Geometry: final body of the model. Coordinates: model frame, mm. A direction names the side the tool comes from. Coordinates: 2 decimals unless noted, no trailing zeros. Order: outer loops, then holes, each group sorted by start corner. A loop starts at its lowest first (then second) coordinate and runs counter-clockwise, first axis right, second up. Notation, with made-up numbers: M 62,0.25 L 72,0.25 A19 ccw 72,14.25 Z; hole C 31,40 d6. An arc over 180 degrees is marked long. One line per question, with ' | ' between items.
from build123d import *

# Parameters (mm, degrees)
SKETCH2_R                 = 23.5
SKETCH2_R_2               = 97
BOSS_EXTRUDE5_DEPTH       = 32
SKETCH3_R                 = 140
SKETCH3_R_2               = 97
BOSS_EXTRUDE8_DEPTH       = 112.5
BOSS_EXTRUDE10_REACH      = 527.627
BOSS_EXTRUDE10_END_RADIUS = 140
SKETCH4_R                 = 100
SKETCH5_R                 = 50
CUT_EXTRUDE1_DEPTH        = 25.5
SKETCH7_R                 = 28.1
CUT_EXTRUDE2_DEPTH        = 328.5
SKETCH9_R                 = 9.714368659
CUT_EXTRUDE3_DEPTH        = 10.5


with BuildPart() as part:
    # Sketch2 → Boss-Extrude5 (new body)
    with BuildSketch(Plane(origin=(0, 0, 0), x_dir=(1, 0, 0), z_dir=(0, 1, 0))):
        with BuildLine():
            ThreePointArc((49.230976904, 178.339293487), (-0.769023096, 228.339293487), (-50.769023096, 178.339293487))
            Line((-50.769023096, 178.339293487), (-50.769023096, 130.470327254))
            ThreePointArc((-50.769023096, 130.470327254), (-121.653121624, 69.285770538), (-138.115414376, -22.893936133))
            Line((-138.115414376, -22.893936133), (-179.061847104, -46.534370091))
            ThreePointArc((-179.061847104, -46.534370091), (-197.363117294, -114.835640281), (-129.061847104, -133.13691047))
            Line((-129.061847104, -133.13691047), (-87.606106294, -109.202427354))
            ThreePointArc((-87.606106294, -109.202427354), (0.823323405, -139.997579045), (88.884437472, -108.164489437))
            Line((88.884437472, -108.164489437), (129.8308702, -131.804923395))
            ThreePointArc((129.8308702, -131.804923395), (198.13214039, -113.503653206), (179.8308702, -45.202383017))
            Line((179.8308702, -45.202383017), (138.37512939, -21.267899901))
            ThreePointArc((138.37512939, -21.267899901), (120.829798219, 70.711808507), (49.230976904, 131.058425571))
            Line((49.230976904, 131.058425571), (49.230976904, 178.339293487))
        make_face()
        with Locations(Location((-0.769023096, 178.339293487, 0), (0, 0, 270))):
            Circle(SKETCH2_R, mode=Mode.SUBTRACT)
        with Locations(Location((0, 0, 0), (0, 0, 270))):
            Circle(SKETCH2_R_2, mode=Mode.SUBTRACT)
        with Locations(Location((-154.061847104, -89.835640281, 0), (0, 0, 270))):
            Circle(SKETCH2_R, mode=Mode.SUBTRACT)
        with Locations(Location((154.8308702, -88.503653206, 0), (0, 0, 270))):
            Circle(SKETCH2_R, mode=Mode.SUBTRACT)
    extrude(amount=BOSS_EXTRUDE5_DEPTH)

    # Sketch3 → Boss-Extrude8 (add)
    with BuildSketch(Plane(origin=(0, 32, 0), x_dir=(1, 0, 0), z_dir=(0, 1, 0))):
        with Locations(Location((0, 0, 0), (0, 0, 69.411740358))):
            Circle(SKETCH3_R)
        with Locations(Location((0, 0, 0), (0, 0, 270))):
            Circle(SKETCH3_R_2, mode=Mode.SUBTRACT)
    extrude(amount=BOSS_EXTRUDE8_DEPTH)

    # Mirror1: part across plane


with BuildPart() as part_1:
    add(part.part)
    add(part.part.mirror(Plane.ZX.offset(144.5)))

    # Boss-Extrude10: up to this cylinder (the profile starts outside it)
    boss_extrude10_end = Plane(origin=(0, 150.900402, 0), z_dir=(0, -1, 0)) * Cylinder(BOSS_EXTRUDE10_END_RADIUS, 1336.254, mode=Mode.PRIVATE)
    # Sketch4 → Boss-Extrude10 (add, up to the surface)
    with BuildSketch(Plane.XY.offset(160), mode=Mode.PRIVATE) as boss_extrude10_sk1:
        with Locations((0, 150.900402454)):
            Circle(SKETCH4_R)
    boss_extrude10_tool1 = extrude(boss_extrude10_sk1.sketch, amount=-BOSS_EXTRUDE10_REACH, mode=Mode.PRIVATE) - boss_extrude10_end
    add(boss_extrude10_tool1.solids().sort_by_distance((0, 150.900402, 160))[0])

    # Sketch5 → Cut-Extrude1 (cut)
    with BuildSketch(Plane.XY.offset(160)):
        with Locations((0, 150.900402454)):
            Circle(SKETCH5_R)
    extrude(amount=-CUT_EXTRUDE1_DEPTH, mode=Mode.SUBTRACT)

    # Sketch7 → Cut-Extrude2 (cut)
    with BuildSketch(Plane.XY.offset(134.5)):
        with Locations(Location((0, 150.900402454, 0), (0, 0, 90))):
            Circle(SKETCH7_R)
    extrude(amount=-CUT_EXTRUDE2_DEPTH, mode=Mode.SUBTRACT)

    # Sketch9 → Cut-Extrude3 (cut)
    with BuildSketch(Plane.XY.offset(160)):
        with Locations((0, 226.895659714)):
            Circle(SKETCH9_R)
        with Locations((65.813823354, 112.902773824)):
            Circle(SKETCH9_R)
        with Locations((-65.813823354, 112.902773824)):
            Circle(SKETCH9_R)
    extrude(amount=-CUT_EXTRUDE3_DEPTH, mode=Mode.SUBTRACT)


solid = part_1.part
1. Access query for faces 1 (the face through (-108.624, 15.776, 121.337)), 2 (the face through (-50.769, 16, -155)), 3 (the face through (-173, 257, 107)), 4 (the face through (133, 32, 79)). Directions: +Z, -Z, +X, -X, +Y, -Y. A direction counts if a zero-diameter tool reaches every point of the face in a straight line with its end or side. Return the directions, or none.
Response values:
face 1: +Z, -Y | face 2: -Z, -X, +Y, -Y | face 3: +Z, -X | face 4: +Z, +X
2. Section A-A, the plane z = 0. Output: boundary loops of the cut face in (x, y), and give its area (3 significant figures).
Response values:
outline: M -140,0 L -97,0 L -97,289 L -140,289 Z; M 97,0 L 140,0 L 140,289 L 97,289 Z | area: 24,900 mm^2
3. Material intervals for line 1 (Y direction, x = 122, z = 96.5); line 2 (X direction, y = 146, z = 105.5); line 3 (X direction, y = 144, z = 106.5), sorted ascending. Write a range as [from, to].
Response values:
line 1: y = [0, 32], [257, 289] | line 2: x = [-99.88, -27.67], [27.67, 99.88] | line 3: x = [-99.76, -27.24], [27.24, 99.76]
4. Section D-D, the plane x = 106. Output: boundary loops of the cut face in (y, z), and give its area (3 significant figures).
Response values:
outline: M 0,-91.45 L 289,-91.45 L 289,118.05 L 257,118.05 L 257,91.45 L 32,91.45 L 32,118.05 L 0,118.05 Z | area: 54,600 mm^2
5. Section B-B, the plane x = -81. Output: boundary loops of the cut face in (y, z).
Response values:
outline: M 0,-114.19 L 289,-114.19 L 289,-53.37 L 0,-53.37 Z; M 0,53.37 L 289,53.37 L 289,114.19 L 209.54,114.19 L 209.54,160 L 92.26,160 L 92.26,114.19 L 0,114.19 Z
6. Section C-C, the plane y = 129. Output: boundary loops of the cut face in (x, z), and give its area (3 significant figures).
Response values:
outline: M -97.57,100.4 A140 ccw -17.61,-138.89 L -17.61,-95.39 A97 cw -17.61,95.39 L -17.61,134.5 L -44.95,134.5 L -44.95,160 L -97.57,160 Z; M 17.61,-138.89 A140 ccw 97.57,100.4 L 97.57,160 L 44.95,160 L 44.95,134.5 L 17.61,134.5 L 17.61,95.39 A97 cw 17.61,-95.39 Z | area: 33,200 mm^2
7. Draft query along X for faces 5 (the face through (0.33, 15.776, -228.327)), 6 (the face through (-1, 257, -202)), 7 (the face through (-130.76, 15.78, 86.78)). Return one class per face: pulls with the +X half, pulls with the -X half, needs draft (parallel to the pull), parting line crosses it, or undercut.
Response values:
face 5: parting line crosses it | face 6: needs draft | face 7: undercut
8. Pin query (flat end, axial travel): P1, Ø1, axis at x = -27.5, y = 250.5, coming from the -Z side; P2, Ø15.5, axis at x = 65.81, y = 112.9, coming from the +Z side; P3, Ø6, axis at x = -101, y = 254.5, coming from the +Z side. Return the tip coordinate at first contact, or that it passes through.
Response values:
P1: stops at z = -137.37 | P2: stops at z = 149.5 | P3: stops at z = 117.89
